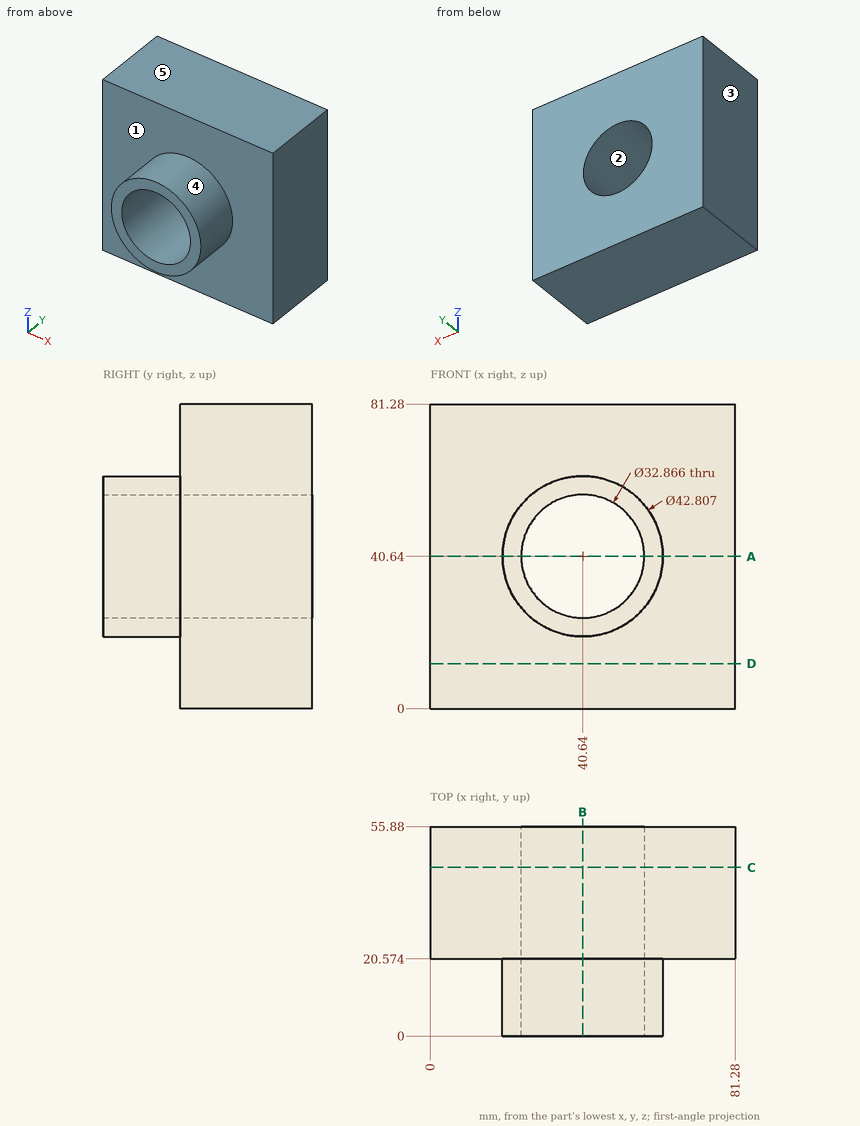
Geometry check sheet. Reference: drawing and pictorial views, mm from the part's lowest x, y, z. A direction names the side the tool comes from. Coordinates: 2 decimals unless noted, no trailing zeros. Loops run counter-clockwise (first coordinate to the right, second up) from the corner with the lowest first, then second, coordinate; pieces in that order, holes last. Notation, with made-up numbers: (-37, 77.25) - (13, 77.25) arc R10 ccw to (13, 86.25) - close; hole circle Ø5 at (13, -11). An arc over 180 degrees is marked (long way). Return JSON: item names as keys, results as strings.
1. Thickness scan on L1, parallel to Z at x = 40.64, y = 11; L2, parallel to Z at x = 40, y = 21; L3, parallel to Y at x = 16.5, z = 19.5. Record the ranges inside material, lowest first.
Established:
{"L1": "z = 19.24 to 24.21, 57.07 to 62.04", "L2": "z = 0 to 24.22, 57.06 to 81.28", "L3": "y = 20.57 to 55.88"}
2. Section check A-A, the plane z = 40.64. Record the boundary of the cut face in (x, y), then the cut area to 3 significant figures.
Established:
{"outline": "(0, 20.57) - (19.24, 20.57) - (19.24, 0) - (24.21, 0) - (24.21, 55.88) - (0, 55.88) - close; (57.07, 0) - (62.04, 0) - (62.04, 20.57) - (81.28, 20.57) - (81.28, 55.88) - (57.07, 55.88) - close", "area": "1,910 mm2"}
3. Tool access check on the marked faces 4 and 5. Record the directions out of +Z, -Z, +X, -X, +Y, -Y that give a thin tool (end or side, any length) a straight path to the whole face; none if there is none.
Established:
{"face 4": "-Y", "face 5": "+Z, +X, -X, +Y, -Y"}
4. Mould release check, pull along X, two halves, no side actions. Record for the marked faces 1, 2 and 3: +X half, -X half, draft (parallel to the pull), parting line (faces both ways), or undercut.
Established:
{"face 1": "draft", "face 2": "undercut", "face 3": "-X half"}
5. Section check D-D, the plane z = 12. Record the boundary of the cut face in (x, y), then the cut area to 3 significant figures.
Established:
{"outline": "(0, 20.57) - (81.28, 20.57) - (81.28, 55.88) - (0, 55.88) - close", "area": "2,870 mm2"}
6. Go/stop test with flat-tipped pins: pin 1 (4 mm diameter, centred on x = 52, y = 8, fed in from +Z); pin 2 (10 mm diameter, centred on x = 20.5, y = 11, fed in from -Z). Record where each tip stops, or that it passes through.
Established:
{"pin 1": "stops at z = 59.89", "pin 2": "stops at z = 25.51"}
7. Section check C-C, the plane y = 45. Record the boundary of the cut face in (x, z) (1 decimal).
Established:
{"outline": "(0, 0) - (81.3, 0) - (81.3, 81.3) - (0, 81.3) - close; hole circle Ø32.9 at (40.6, 40.6)"}
8. Section check B-B, the plane x = 40.64. Record the boundary of the cut face in (y, z).
Established:
{"outline": "(0, 19.24) - (20.57, 19.24) - (20.57, 0) - (55.88, 0) - (55.88, 24.21) - (0, 24.21) - close; (0, 57.07) - (55.88, 57.07) - (55.88, 81.28) - (20.57, 81.28) - (20.57, 62.04) - (0, 62.04) - close"}
